Can you work these out from the model? Positions are in its coordinate system, mm. Face numbers are marked on the shaded views. A direction names the side the tool comes from. Round coordinates to 2 decimals unless told otherwise and drop trailing zeros. Order: outer loops, then holes, each group sorted by start corner. A loop starts at its lowest first (then second) coordinate and runs counter-clockwise, first axis right, second up. Notation, with made-up numbers: M 57.5,56 L 102.5,56 A19 ccw 102.5,82 Z; hole C 47,1.25 d7. An arc over 180 degrees is marked long. One line per question, with ' | ' between items.
```python
from build123d import *

# Parameters (mm, degrees)
BOSS_EXTRUDE1_DEPTH = 10
SKETCH2_R           = 1.85
CUT_EXTRUDE1_DEPTH  = 19.547236991
SKETCH4_R           = 1.7
CUT_EXTRUDE2_DEPTH  = 19.547236991
CUT_EXTRUDE3_DEPTH  = 2.5


with BuildPart() as part:
    # Sketch1 → Boss-Extrude1 (new body)
    with BuildSketch(Plane(origin=(0, 0, 0), x_dir=(0, 0, -1), z_dir=(1, 0, 0))):
        Polygon((-5, 12), (0, 12), (0, 0), (10, 0), (10, -3), (-5, -3), align=None)
    extrude(amount=BOSS_EXTRUDE1_DEPTH)

    # Sketch2 → Cut-Extrude1 (cut, through all)
    with BuildSketch(Plane(origin=(0, 0, 0), x_dir=(1, 0, 0), z_dir=(0, 1, 0))):
        with Locations(Location((5, 5, 0), (0, 0, 270))):
            Circle(SKETCH2_R)
    extrude(amount=-CUT_EXTRUDE1_DEPTH, mode=Mode.SUBTRACT)

    # Sketch4 → Cut-Extrude2 (cut, through all)
    with BuildSketch(Plane(origin=(0, 0, 0), x_dir=(-1, 0, 0), z_dir=(0, 0, -1))):
        with Locations((-5, 6)):
            Circle(SKETCH4_R)
    extrude(amount=-CUT_EXTRUDE2_DEPTH, mode=Mode.SUBTRACT)

    # Sketch5 → Cut-Extrude3 (cut)
    with BuildSketch(Plane(origin=(0, 0, 0), x_dir=(-1, 0, 0), z_dir=(0, 0, -1))):
        Polygon((-3.325684219, 3.1), (-1.651368439, 6), (-3.325684219, 8.9), (-6.674315781, 8.9), (-8.348631561, 6), (-6.674315781, 3.1), align=None)
    extrude(amount=-CUT_EXTRUDE3_DEPTH, mode=Mode.SUBTRACT)


solid = part.part
```
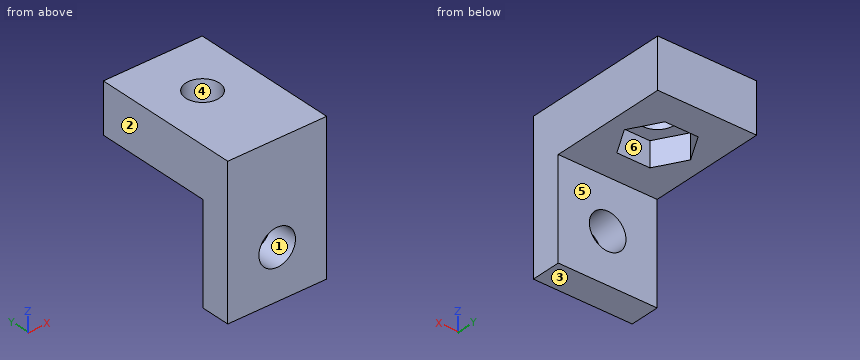
(1) Thinking about a two-plate mould opening in Z: for the marked faces 1, 2 and 3, which applies, released by +Z, released by -Z, zero draft, split by the parting line, or undercut?
Final values:
face 1: undercut | face 2: zero draft | face 3: released by -Z
(2) If we section it at B-B on y = 4.75: Please give me the cut outline in (x, z), plus the area to 3 significant figures.
Final values:
outline: M 0,0 L 2.37,0 L 2.37,2.5 L 3.85,2.5 L 3.85,5 L 0,5 Z; M 6.15,2.5 L 7.63,2.5 L 7.63,0 L 10,0 L 10,5 L 6.15,5 Z | area: 31.1 mm^2
(3) On a 3-axis mill with a long thin cutter (end or side, diameter ignored), from which of +Z, -Z, +X, -X, +Y, -Y can I reach the whole of each face in a straight line? I mean the marked faces 4, 5 and 6. Say none if no direction works.
Final values:
face 4: +Z, -Z | face 5: -Z, +X, -X, +Y | face 6: -Z
(4) Please list where these lines run through material, in increasing order: probe 1 along Y at (x, z) = (5, 4.05); probe 2 along Z at (x, y) = (3.5, 10.75); probe 3 along Z at (x, y) = (2, 6.25). Write a range as [from, to].
Final values:
probe 1: [-3, 4.3], [7.7, 12] | probe 2: [0, 5] | probe 3: [2.5, 5]
(5) If we section it at A-A on x = 5: Please give me the cut outline in (y, z), plus the area to 3 significant figures.
Final values:
outline: M -3,-10 L 0,-10 L 0,-6.85 L -3,-6.85 Z; M -3,-3.15 L 0,-3.15 L 0,0 L 3.1,0 L 3.1,2.5 L 4.3,2.5 L 4.3,5 L -3,5 Z; M 7.7,2.5 L 8.9,2.5 L 8.9,0 L 12,0 L 12,5 L 7.7,5 Z | area: 70.9 mm^2
(6) If we section it at D-D on y = -1.75: Please give me the cut outline in (x, z).
Final values:
outline: M 0,-10 L 10,-10 L 10,5 L 0,5 Z; hole C 5,-5 d3.7
(7) Will these pins go through, and if not, where does the flat tip stop? pin 1 Ø5 at (x, y) = (3.5, 4.5) entering from -Z; pin 2 Ø4 at (x, y) = (5, 6) entering from -Z.
Final values:
pin 1: z = 0 | pin 2: z = 2.5
(8) If we section it at C-C on z = 1.5: Please give me the cut outline in (x, y), plus the area to 3 significant figures.
Final values:
outline: M 0,-3 L 10,-3 L 10,12 L 0,12 Z; hole M 1.65,6 L 3.33,3.1 L 6.67,3.1 L 8.35,6 L 6.67,8.9 L 3.33,8.9 Z | area: 121 mm^2
